```python
from build123d import *

# Parameters (mm, degrees)
SKETCH4_R           = 75
SKETCH4_R_2         = 9.65
SKETCH4_R_3         = 2
SKETCH4_R_4         = 7.65
BOSS_EXTRUDE1_DEPTH = 5.5


with BuildPart() as part:
    # Sketch4 → Boss-Extrude1 (new body)
    with BuildSketch(Plane(origin=(0, 0, 0), x_dir=(1, 0, 0), z_dir=(0, 1, 0))):
        with Locations(Location((0, 0, 0), (0, 0, 270))):
            Circle(SKETCH4_R)
        with Locations(Location((-36.827392181, 0, 0), (0, 0, 270))):
            Circle(SKETCH4_R_2, mode=Mode.SUBTRACT)
        with Locations(Location((-18.413696091, 31.893457184, 0), (0, 0, 270))):
            Circle(SKETCH4_R_2, mode=Mode.SUBTRACT)
        with Locations(Location((18.413696091, 31.893457184, 0), (0, 0, 270))):
            Circle(SKETCH4_R_2, mode=Mode.SUBTRACT)
        with Locations(Location((36.827392181, 0, 0), (0, 0, 270))):
            Circle(SKETCH4_R_2, mode=Mode.SUBTRACT)
        with Locations(Location((18.413696091, -31.893457184, 0), (0, 0, 270))):
            Circle(SKETCH4_R_2, mode=Mode.SUBTRACT)
        with Locations(Location((-18.413696091, -31.893457184, 0), (0, 0, 270))):
            Circle(SKETCH4_R_2, mode=Mode.SUBTRACT)
        with Locations(Location((0, 13.5, 0), (0, 0, 270))):
            Circle(SKETCH4_R_3, mode=Mode.SUBTRACT)
        with Locations(Location((11.691342951, 6.75, 0), (0, 0, 270))):
            Circle(SKETCH4_R_3, mode=Mode.SUBTRACT)
        with Locations(Location((11.691342951, -6.75, 0), (0, 0, 270))):
            Circle(SKETCH4_R_3, mode=Mode.SUBTRACT)
        with Locations(Location((0, -13.5, 0), (0, 0, 270))):
            Circle(SKETCH4_R_3, mode=Mode.SUBTRACT)
        with Locations(Location((-11.691342951, -6.75, 0), (0, 0, 270))):
            Circle(SKETCH4_R_3, mode=Mode.SUBTRACT)
        with Locations(Location((-11.691342951, 6.75, 0), (0, 0, 270))):
            Circle(SKETCH4_R_3, mode=Mode.SUBTRACT)
        with Locations(Location((0, 55, 0), (0, 0, 270))):
            Circle(SKETCH4_R_4, mode=Mode.SUBTRACT)
        with Locations(Location((47.631397208, -27.5, 0), (0, 0, 270))):
            Circle(SKETCH4_R_4, mode=Mode.SUBTRACT)
        with Locations(Location((-47.631397208, -27.5, 0), (0, 0, 270))):
            Circle(SKETCH4_R_4, mode=Mode.SUBTRACT)
        with Locations(Location((37.979389645, -37.152007563, 0), (0, 0, 270))):
            Circle(SKETCH4_R_3, mode=Mode.SUBTRACT)
        with Locations(Location((37.979389645, -17.847992437, 0), (0, 0, 270))):
            Circle(SKETCH4_R_3, mode=Mode.SUBTRACT)
        with Locations(Location((57.283404771, -17.847992437, 0), (0, 0, 270))):
            Circle(SKETCH4_R_3, mode=Mode.SUBTRACT)
        with Locations(Location((57.283404771, -37.152007563, 0), (0, 0, 270))):
            Circle(SKETCH4_R_3, mode=Mode.SUBTRACT)
        with Locations(Location((-51.164277174, -14.315112471, 0), (0, 0, 270))):
            Circle(SKETCH4_R_3, mode=Mode.SUBTRACT)
        with Locations(Location((-60.816284737, -31.032879966, 0), (0, 0, 270))):
            Circle(SKETCH4_R_3, mode=Mode.SUBTRACT)
        with Locations(Location((-44.098517242, -40.684887529, 0), (0, 0, 270))):
            Circle(SKETCH4_R_3, mode=Mode.SUBTRACT)
        with Locations(Location((-34.446509679, -23.967120034, 0), (0, 0, 270))):
            Circle(SKETCH4_R_3, mode=Mode.SUBTRACT)
        with Locations(Location((13.184887529, 51.467120034, 0), (0, 0, 270))):
            Circle(SKETCH4_R_3, mode=Mode.SUBTRACT)
        with Locations(Location((3.532879966, 68.184887529, 0), (0, 0, 270))):
            Circle(SKETCH4_R_3, mode=Mode.SUBTRACT)
        with Locations(Location((-13.184887529, 58.532879966, 0), (0, 0, 270))):
            Circle(SKETCH4_R_3, mode=Mode.SUBTRACT)
        with Locations(Location((-3.532879966, 41.815112471, 0), (0, 0, 270))):
            Circle(SKETCH4_R_3, mode=Mode.SUBTRACT)
        Polygon((3.75277675, -6.5), (7.505553499, 0), (3.75277675, 6.5), (-3.75277675, 6.5), (-7.505553499, 0), (-3.75277675, -6.5), align=None, mode=Mode.SUBTRACT)
    extrude(amount=BOSS_EXTRUDE1_DEPTH)


solid = part.part
```
Could you check a few things on this model? Use its own coordinates, in mm. Round coordinates to 2 decimals unless told otherwise and drop trailing zeros. Loops run counter-clockwise (first coordinate to the right, second up) from the corner with the lowest first, then second, coordinate; pieces in that order, holes last.
Q1. I want a section at B-B (x = -21.5). Write out the boundary of the cut face in (y, z), and give its area (3 significant figures).
Q2. I want a section at A-A (z = -13.5). Write out the boundary of the cut face in (x, y) (3 decimals), and give its area (3 significant figures).
Q3. For P1, Ø2, axis at x = -51.5, y = 3, coming from the +Z side; P2, Ø3, axis at x = 11.69, z = -6.75, coming from the -Y side; P3, Ø2, axis at x = -48, y = 1.5, coming from the +Z side; P4, Ø3, axis at x = 23.5, y = 2.5, coming from the -Z side, each with a flat end and sliding along its axis, tell me the tip position at first contact or that it passes through.
Q4. Thinking about a two-plate mould opening in X: for faces 1 (the flat face through (-16, 5.5, -1)), 2 (the cylindrical face through (-44.865, 2.712, 42.532)), which applies, pulls with the +X half, pulls with the -X half, needs draft (parallel to the pull), parting line crosses it, or undercut?
Q5. I want a section at C-C (y = 2.25). Give the number of separate pieces and of enclosed holes in the cut face, and give its area (3 significant figures).
Q6. I want a section at D-D (z = 58.5). Write out the boundary of the cut face in (x, y), and give its area (3 significant figures).
Q7. Please list where these lines run through material, in increasing order: L1, parallel to X at y = 3.8, z = 0; L2, parallel to Z at x = 58, y = 3.1; L3, parallel to X at y = 3.65, z = 38.5.
Answer below:
1. outline: (0, -71.85) - (5.5, -71.85) - (5.5, -41.04) - (0, -41.04) - close; (0, -22.75) - (5.5, -22.75) - (5.5, 22.75) - (0, 22.75) - close; (0, 41.04) - (5.5, 41.04) - (5.5, 71.85) - (0, 71.85) - close
1. area: 589 mm2
2. outline: (-73.775, 0) - (-2, 0) - (-2, 5.5) - (-73.775, 5.5) - close; (2, 0) - (73.775, 0) - (73.775, 5.5) - (2, 5.5) - close
2. area: 790 mm2
3. P1: stops at z = 55.45
3. P2: passes through
3. P3: stops at z = 58.45
3. P4: stops at z = -71.7
4. face 1: needs draft
4. face 2: undercut
5. separate pieces: 1
5. enclosed holes: 28
5. area: 15,000 mm2
6. outline: (-46.93, 0) - (46.93, 0) - (46.93, 5.5) - (-46.93, 5.5) - close
6. area: 516 mm2
7. L1: x = -75 to -46.48, -27.18 to -7.51, 7.51 to 27.18, 46.48 to 75
7. L2: z = -47.55 to 15.98, 19.72 to 35.28, 39.02 to 47.55
7. L3: x = -64.36 to -25.45, -11.38 to 11.38, 25.45 to 36.5, 39.46 to 55.81, 58.76 to 64.36
